from build123d import *

# Parameters (mm, degrees)
SKETCH1_W                = 34.714871787
SKETCH1_H                = 10.923666426
BOSS_EXTRUDE1_DEPTH      = 1
BOSS_EXTRUDE2_DEPTH      = 11
BOSS_EXTRUDE3_DEPTH      = 5
BOSS_EXTRUDE3_DEPTH_BACK = 3
SKETCH3_W                = 50
SKETCH3_H                = 7
CUT_EXTRUDE3_DEPTH       = 25
SKETCH5_W                = 50
SKETCH5_H                = 7
CUT_EXTRUDE4_DEPTH       = 25
SKETCH6_W                = 50
SKETCH6_H                = 7
CUT_EXTRUDE5_DEPTH       = 25
SKETCH8_R                = 1.5
BOSS_EXTRUDE5_DEPTH      = 1
BOSS_EXTRUDE10_DEPTH     = 3


with BuildPart() as part:
    # Sketch1 → Boss-Extrude1 (new body)
    with BuildSketch(Plane(origin=(0, 0, 0), x_dir=(1, 0, 0), z_dir=(0, 1, 0))):
        Polygon((243.304219775, -116.484791865), (254.809280577, -136.408896137), (442.602090749, -136.409305398), (444.621046679, -132.925433224), (441.749040748, -132.925433224), (449.516726724, -119.471406458), (450.964695298, -121.978953123), (452.699916622, -118.984688018), (358.778179036, 43.666038065), (335.767496284, 43.666038065), align=None)
        with Locations((422.370878913, -129.522754792)):
            Rectangle(SKETCH1_W, SKETCH1_H, mode=Mode.SUBTRACT)
        Polygon((423.190377512, -92.577472767), (432.651287025, -87.114324326), (450.119365975, -117.364996826), (440.658456462, -122.828145267), align=None, mode=Mode.SUBTRACT)
        Polygon((428.113670919, -116.417164681), (266.439108268, -116.428009237), (347.273609729, 23.609230821), align=None, mode=Mode.SUBTRACT)
    extrude(amount=BOSS_EXTRUDE1_DEPTH)

    # Sketch1_9 → Boss-Extrude2 (add)
    # profile 1 of 2: a face of its own
    with BuildSketch(Plane(origin=(0, 0, 0), x_dir=(1, 0, 0), z_dir=(0, 1, 0))):
        Polygon((229.159432548, -134.984249184), (231.716666588, -139.412373829), (462.829865412, -139.412373829), (465.38624875, -134.984588004), (349.829542096, 65.165499075), (344.716133219, 65.165499075), align=None)
        Polygon((251.922647989, -136.409305399), (233.446303401, -136.408896138), (232.62355396, -134.984217357), (241.860901689, -118.984688018), align=None, mode=Mode.SUBTRACT)
        Polygon((442.602090749, -136.409305398), (254.809280577, -136.408896137), (243.304219775, -116.484791865), (335.767496284, 43.666038065), (358.778179036, 43.666038065), (461.938967958, -134.984588006), (461.116393749, -136.409305398), align=None, mode=Mode.SUBTRACT)
        Polygon((348.096628302, 62.164013367), (357.334800991, 46.166038067), (337.210874326, 46.166038067), (346.44844193, 62.165948237), align=None, mode=Mode.SUBTRACT)
    # profile 2 of 2: a face of its own
    with BuildSketch(Plane(origin=(0, 0, 0), x_dir=(1, 0, 0), z_dir=(0, 1, 0))):
        Polygon((441.749040748, -132.925433224), (444.621046679, -132.925433224), (450.964695298, -121.978953123), (449.516726724, -119.471406458), align=None)
    extrude(amount=BOSS_EXTRUDE2_DEPTH)

    # Sketch1_10 → Boss-Extrude3 (add, two sides: drawn at the far end of the back side and taken through both)
    # profile 1 of 2: a face of its own
    with BuildSketch(Plane(origin=(0, 0, 0), x_dir=(1, 0, 0), z_dir=(0, 1, 0)).offset(-BOSS_EXTRUDE3_DEPTH_BACK)):
        Polygon((229.159432548, -134.984249184), (231.716666588, -139.412373829), (462.829865412, -139.412373829), (465.38624875, -134.984588004), (349.829542096, 65.165499075), (344.716133219, 65.165499075), align=None)
        Polygon((251.922647989, -136.409305399), (233.446303401, -136.408896138), (232.62355396, -134.984217357), (241.860901689, -118.984688018), align=None, mode=Mode.SUBTRACT)
        Polygon((442.602090749, -136.409305398), (254.809280577, -136.408896137), (243.304219775, -116.484791865), (335.767496284, 43.666038065), (358.778179036, 43.666038065), (461.938967958, -134.984588006), (461.116393749, -136.409305398), align=None, mode=Mode.SUBTRACT)
        Polygon((348.096628302, 62.164013367), (357.334800991, 46.166038067), (337.210874326, 46.166038067), (346.44844193, 62.165948237), align=None, mode=Mode.SUBTRACT)
    # profile 2 of 2: a face of its own
    with BuildSketch(Plane(origin=(0, 0, 0), x_dir=(1, 0, 0), z_dir=(0, 1, 0)).offset(-BOSS_EXTRUDE3_DEPTH_BACK)):
        Polygon((441.749040748, -132.925433224), (444.621046679, -132.925433224), (450.964695298, -121.978953123), (449.516726724, -119.471406458), align=None)
    extrude(amount=BOSS_EXTRUDE3_DEPTH + BOSS_EXTRUDE3_DEPTH_BACK)

    # Sketch3 → Cut-Extrude3 (cut)
    with BuildSketch(Plane(origin=(290.589645397, 0, -167.772009994), x_dir=(-0.49999999999998745, 0, -0.8660254037844459), z_dir=(0.8660254037844459, 0, -0.49999999999998745))):
        with Locations((-236.592990632, -3)):
            Rectangle(SKETCH3_W, SKETCH3_H)
    extrude(amount=-CUT_EXTRUDE3_DEPTH, mode=Mode.SUBTRACT)

    # Sketch5 → Cut-Extrude4 (cut)
    with BuildSketch(Plane.XY.offset(139.412373829)):
        with Locations((347.273266, -3)):
            Rectangle(SKETCH5_W, SKETCH5_H)
    extrude(amount=-CUT_EXTRUDE4_DEPTH, mode=Mode.SUBTRACT)

    # Sketch6 → Cut-Extrude5 (cut)
    with BuildSketch(Plane(origin=(230.319375798, 0, 132.975171837), x_dir=(-0.5000006154012504, 0, 0.8660250484820695), z_dir=(-0.8660250484820695, 0, -0.5000006154012504))):
        with Locations((-113.236674799, -3)):
            Rectangle(SKETCH6_W, SKETCH6_H)
    extrude(amount=-CUT_EXTRUDE5_DEPTH, mode=Mode.SUBTRACT)

    # Sketch8 → Boss-Extrude5 (add)
    with BuildSketch(Plane.XZ.offset(3)):
        Polygon((349.829542096, -65.165499075), (465.38624875, 134.984588004), (462.829865412, 139.412373829), (231.716666588, 139.412373829), (229.159432548, 134.984249184), (344.716133219, -65.165499075), align=None)
        with Locations(Location((395.323540807, 98.692824234, 0), (0, 0, 270))):
            Circle(SKETCH8_R, mode=Mode.SUBTRACT)
        with Locations(Location((348.301285091, 15.863526629, 0), (0, 0, 270))):
            Circle(SKETCH8_R, mode=Mode.SUBTRACT)
        with Locations(Location((299.654911442, 97.24168178, 0), (0, 0, 270))):
            Circle(SKETCH8_R, mode=Mode.SUBTRACT)
        Polygon((414.793175166, 116.418058172), (444.621046679, 132.925433224), (450.964695298, 121.978953123), (423.743256024, 108.846989255), (416.453113266, 96.21943309), (438.086080689, 105.056150836), (452.699916622, 118.984688018), (461.938967958, 134.984588006), (461.116393749, 136.409305398), (442.602090749, 136.409305398), (432.302823198, 135.574995335), (404.013141868, 116.418781259), align=None, mode=Mode.SUBTRACT)
        Polygon((322.273266, 116.42426408), (294.358218631, 68.061097964), (319.354499367, 24.757680453), (376.473657316, 26.969372806), (401.47267951, 70.271207531), (372.273266, 116.420910257), align=None, mode=Mode.SUBTRACT)
        Polygon((233.446303401, 136.408896138), (251.922647989, 136.409305399), (241.860901689, 118.984688018), (232.62355396, 134.984217357), align=None, mode=Mode.SUBTRACT)
        Polygon((337.210874326, -46.166038067), (357.334800991, -46.166038067), (348.096628302, -62.164013367), (346.44844193, -62.165948237), align=None, mode=Mode.SUBTRACT)
        Polygon((418.423760883, 112.300563217), (412.029962691, 98.692824234), (402.084054392, 110.169297153), align=None, mode=Mode.SUBTRACT)
    extrude(amount=BOSS_EXTRUDE5_DEPTH)

    # Sketch12 → Boss-Extrude10 (add)
    with BuildSketch(Plane(origin=(0, -3, 0), x_dir=(1, 0, 0), z_dir=(0, 1, 0))):
        with BuildLine():
            Line((347.417900211, -11.962292061), (347.307477101, -11.47463774))
            ThreePointArc((347.307477101, -11.47463774), (345.119304576, -12.681546114), (343.912396202, -14.869718639))
            Line((343.912396203, -14.869718639), (344.400050524, -14.980141749))
            ThreePointArc((344.400050523, -14.980141749), (345.472857967, -13.035099504), (347.417900211, -11.962292061))
        make_face()
        with BuildLine():
            ThreePointArc((352.690173981, -14.869718639), (351.483265607, -12.681546114), (349.295093082, -11.47463774))
            Line((349.295093081, -11.47463774), (349.184669971, -11.962292061))
            ThreePointArc((349.184669972, -11.962292061), (351.129712216, -13.035099504), (352.20251966, -14.980141749))
            Line((352.202519659, -14.980141749), (352.69017398, -14.869718639))
        make_face()
        with BuildLine():
            ThreePointArc((349.295093082, -20.252415518), (351.483265607, -19.045507145), (352.690173981, -16.857334619))
            Line((352.69017398, -16.857334619), (352.202519659, -16.746911509))
            ThreePointArc((352.20251966, -16.746911509), (351.129712216, -18.691953754), (349.184669972, -19.764761197))
            Line((349.184669971, -19.764761197), (349.295093081, -20.252415518))
        make_face()
        with BuildLine():
            Line((344.400050524, -16.746911509), (343.912396203, -16.857334619))
            ThreePointArc((343.912396202, -16.857334619), (345.119304576, -19.045507145), (347.307477101, -20.252415518))
            Line((347.307477101, -20.252415518), (347.417900211, -19.764761197))
            ThreePointArc((347.417900211, -19.764761197), (345.472857967, -18.691953754), (344.400050523, -16.746911509))
        make_face()
        with BuildLine():
            Line((394.440155927, -94.791589666), (394.329732817, -94.303935345))
            ThreePointArc((394.329732817, -94.303935345), (392.141560292, -95.510843718), (390.934651918, -97.699016244))
            Line((390.934651918, -97.699016244), (391.4247896, -97.798542945))
            ThreePointArc((391.4247896, -97.798542945), (392.499067689, -95.860448622), (394.440155927, -94.791589666))
        make_face()
        with BuildLine():
            ThreePointArc((399.712429696, -97.699016244), (398.505521323, -95.510843718), (396.317348797, -94.303935345))
            Line((396.317348797, -94.303935345), (396.206925687, -94.791589666))
            ThreePointArc((396.206925687, -94.791589666), (398.151967932, -95.864397109), (399.224775375, -97.809439354))
            Line((399.224775375, -97.809439354), (399.712429696, -97.699016244))
        make_face()
        with BuildLine():
            ThreePointArc((396.317348797, -103.081713123), (398.505521323, -101.874804749), (399.712429696, -99.686632224))
            Line((399.712429696, -99.686632224), (399.224775375, -99.576209114))
            ThreePointArc((399.224775375, -99.576209114), (398.151967932, -101.521251358), (396.206925687, -102.594058802))
            Line((396.206925687, -102.594058801), (396.317348797, -103.081713122))
        make_face()
        with BuildLine():
            Line((391.422306239, -99.576209114), (390.934651918, -99.686632224))
            ThreePointArc((390.934651918, -99.686632224), (392.141560292, -101.874804749), (394.329732817, -103.081713123))
            Line((394.329732817, -103.081713122), (394.440155927, -102.594058801))
            ThreePointArc((394.440155927, -102.594058802), (392.495113682, -101.521251358), (391.422306239, -99.576209114))
        make_face()
        with BuildLine():
            ThreePointArc((298.661103452, -92.852792892), (296.472930927, -94.059701265), (295.266022553, -96.24787379))
            Line((295.266022553, -96.24787379), (295.753676874, -96.3582969))
            ThreePointArc((295.753676874, -96.3582969), (296.826484317, -94.413254656), (298.771526562, -93.340447213))
            Line((298.771526562, -93.340447212), (298.661103452, -92.852792891))
        make_face()
        with BuildLine():
            ThreePointArc((304.04380033, -96.24787379), (302.836891957, -94.059701265), (300.648719432, -92.852792892))
            Line((300.648719432, -92.852792891), (300.538296322, -93.340447212))
            ThreePointArc((300.538296322, -93.340447213), (302.483338566, -94.413254656), (303.55614601, -96.3582969))
            Line((303.55614601, -96.3582969), (304.043800331, -96.24787379))
        make_face()
        with BuildLine():
            Line((300.538296322, -101.142916348), (300.648719432, -101.630570669))
            ThreePointArc((300.648719432, -101.630570669), (302.836891957, -100.423662295), (304.04380033, -98.23548977))
            Line((304.043800331, -98.23548977), (303.55614601, -98.12506666))
            ThreePointArc((303.55614601, -98.12506666), (302.483338566, -100.070108905), (300.538296322, -101.142916348))
        make_face()
        with BuildLine():
            Line((295.753676874, -98.12506666), (295.266022553, -98.23548977))
            ThreePointArc((295.266022553, -98.23548977), (296.472930927, -100.423662295), (298.661103452, -101.630570669))
            Line((298.661103452, -101.630570669), (298.771526562, -101.142916348))
            ThreePointArc((298.771526562, -101.142916348), (296.826484317, -100.070108905), (295.753676874, -98.12506666))
        make_face()
    extrude(amount=BOSS_EXTRUDE10_DEPTH)


solid = part.part
Check sheet for the modelled part. Datum: model origin and axes. Units: mm. A direction names the side the tool comes from. Round coordinates to 2 decimals unless told otherwise and drop trailing zeros. Loops run counter-clockwise (first coordinate to the right, second up) from the corner with the lowest first, then second, coordinate; pieces in that order, holes last. Notation, with made-up numbers: M 84,-14.75 L 128,-14.75 A17 ccw 128,-6.75 Z; hole C 62.5,6.25 d5. An arc over 180 degrees is marked long. One line per question, with ' | ' between items. Start each with the question number.
Item 1: Section check B-B (z = 90). Record the boundary of the cut face in (x, y), and give its area (3 significant figures).
Item 2: Set-up check for faces 1 (the face through (347, 6, -43.666)), 2 (the face through (237.31, 3.61, 126.87)), 3 (the face through (297, 0.5, 40)): record each of +Z, -Z, +X, -X, +Y, -Y from which the full face is reachable in a straight line by a thin tool's end or side.
Item 3: Section check D-D (z = -51.5). Record the boundary of the cut face in (x, y).
Item 4: Section check A-A (y = 6). Record the boundary of the cut face in (x, z).
Item 5: Scan lines: probe 1 along Y at (x, z) = (321, 124.5); probe 2 along Z at (x, y) = (447, 6.25); probe 3 along X at (y, z) = (6, 121). Record each from-to range of solid material in increasing order.
Item 6: Gauge pin test, flat ends, axial feed: pin 1 Ø3 at (x, z) = (343.5, 114) entering from +Y; pin 2 Ø5 at (x, y) = (299, 7) entering from -Z; pin 3 Ø1.1 at (x, y) = (424.5, 0.5) entering from -Z; pin 4 Ø4 at (x, z) = (398, 96) entering from +Y. Record the tip position at first contact, or that the pin passes through.
Item 7: Section check C-C (x = 285.5). Record the boundary of the cut face in (y, z), and give its area (3 significant figures).
Item 8: Release check for a two-part mould opening along X. For faces 4 (the face through (376.04, -1.52, -13.77)), 5 (the face through (408, 11, 37)), 6 (the face through (406.8, 3.61, 33.51)) record: released by +X, released by -X, zero draft, split by the parting line, or undercut.
Worked out:
1) outline: M 255.13,-4 L 307.02,-4 L 307.02,-3 L 258.6,-3 L 258.6,0 L 281.69,0 L 281.69,1 L 258.6,1 L 258.6,11 L 255.13,11 Z; M 388.99,-4 L 439.41,-4 L 439.41,11 L 435.96,11 L 435.96,1 L 434.32,1 L 434.32,0 L 435.96,0 L 435.96,-3 L 388.99,-3 Z; M 412.86,0 L 427.65,0 L 427.65,1 L 412.86,1 Z | area: 239 mm^2
2) face 1: +Y | face 2: +Y, -Y | face 3: none
3) outline: M 336.83,-4 L 340.29,-4 L 340.29,11 L 336.83,11 Z; M 354.25,-4 L 357.72,-4 L 357.72,11 L 354.25,11 Z
4) outline: M 229.16,134.98 L 344.72,-65.17 L 349.83,-65.17 L 465.39,134.98 L 462.83,139.41 L 231.72,139.41 Z; M 441.75,132.93 L 449.52,119.47 L 450.96,121.98 L 444.62,132.93 Z; hole M 232.62,134.98 L 241.86,118.98 L 251.92,136.41 L 233.45,136.41 Z; hole M 243.3,116.48 L 335.77,-43.67 L 358.78,-43.67 L 461.94,134.98 L 461.12,136.41 L 442.6,136.41 L 254.81,136.41 Z; hole M 337.21,-46.17 L 346.45,-62.17 L 348.1,-62.16 L 357.33,-46.17 Z
5) probe 1: -4 to -3, 0 to 1 | probe 2: 103.14 to 109.11, 123.83 to 128.82, 136.41 to 139.41 | probe 3: 237.23 to 240.7, 243.02 to 245.91, 448.63 to 450.4, 453.86 to 457.31
6) pin 1: through | pin 2: z = 9.69 | pin 3: z = 63.21 | pin 4: y = 0
7) outline: M -4,37.4 L -3,37.4 L -3,136.41 L 0,136.41 L 0,116.43 L 1,116.43 L 1,136.41 L 11,136.41 L 11,139.41 L -4,139.41 Z; M 0,62.95 L 0.5,62.95 L 0.5,37.4 L 11,37.4 L 11,43.4 L 1,43.4 L 1,83.41 L 0,83.41 Z | area: 257 mm^2
8) face 4: undercut | face 5: zero draft | face 6: released by +X
